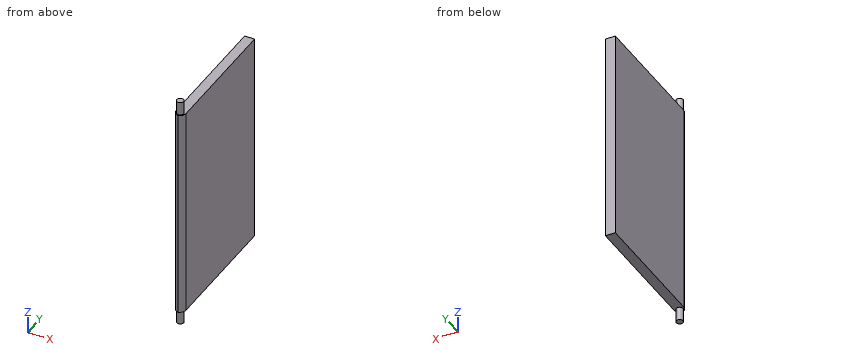
```python
from build123d import *

# Parameters (mm, degrees)
SKETCH1_W           = 101.6
SKETCH1_H           = 64.682803082
BOSS_EXTRUDE1_DEPTH = 4.7625
SKETCH2_R           = 1.631191497
BOSS_EXTRUDE2_DEPTH = 6.35
FILLET2_R           = 3.175


with BuildPart() as part:
    # Sketch1 → Boss-Extrude1 (new body)
    with BuildSketch(Plane(origin=(0, 0, 0), x_dir=(0, 0, -1), z_dir=(1, 0, 0))):
        with Locations((0, 26.994954374)):
            Rectangle(SKETCH1_W, SKETCH1_H)
    extrude(amount=-BOSS_EXTRUDE1_DEPTH)

    # Sketch2 → Boss-Extrude2 (add)
    with BuildSketch(Plane.XY.offset(50.8)):
        with Locations((-2.38125, -2.965197167)):
            Circle(SKETCH2_R)
    boss_extrude2 = extrude(amount=BOSS_EXTRUDE2_DEPTH)

    # Mirror1: Boss-Extrude2 across plane
    add(boss_extrude2.mirror(Plane.XY))

    # Fillet2
    # the kernel refuses this fillet: 3.175 mm, written as the material it takes off along each edge
    with BuildSketch(Plane(origin=(0, -5.346447167, 58.7375), x_dir=(0, 1, 0), z_dir=(0, 0, -1))) as fillet2_piece_1:
        with BuildLine():
            CenterArc((FILLET2_R, -FILLET2_R), FILLET2_R, 90, 90)
            Line((0, -FILLET2_R), (0, 0))
            Line((0, 0), (FILLET2_R, 0))
        make_face()
    extrude(amount=117.475, mode=Mode.SUBTRACT)
    with BuildSketch(Plane(origin=(-4.7625, -5.346447167, 58.7375), x_dir=(0, 1, 0), z_dir=(0, 0, -1))) as fillet2_piece_2:
        with BuildLine():
            CenterArc((FILLET2_R, FILLET2_R), FILLET2_R, 180, 90)
            Line((0, FILLET2_R), (0, 0))
            Line((0, 0), (FILLET2_R, 0))
        make_face()
    extrude(amount=117.475, mode=Mode.SUBTRACT)


solid = part.part
```
Could you check a few things on this model? Use its own coordinates, in mm. Give positions to 0.01 mm unless a question says otherwise; leave off trailing zeros. Order: outer loops, then holes, each group sorted by start corner. A loop starts at its lowest first (then second) coordinate and runs counter-clockwise, first axis right, second up.
Q1. Suppose I cut it at A-A, the plane y = 25. Write out the boundary of the cut face in (x, z).
Q2. Suppose I cut it at B-B, the plane x = -3.1. Write out the boundary of the cut face in (y, z).
Q3. I'm going to push a flat-ended pin straight in: P1, Ø1.5, axis at x = -2, y = 47.5, coming from the -Z side. Where does the tip first touch, or does it pass through?
Q4. If I drill on line 1 along Z through (x, y) = (-1.9, 48.5); line 2 along Y through (x, z) = (-2.3, -33.5); line 3 along Y through (x, z) = (-3.7, 8), over which ranges is the centre line in solid material (lowest first)?
Solution:
1. outline: (-4.76, -50.8) - (0, -50.8) - (0, 50.8) - (-4.76, 50.8) - close
2. outline: (-4.96, -50.8) - (-4.43, -50.8) - (-4.43, -57.15) - (-1.5, -57.15) - (-1.5, -50.8) - (59.34, -50.8) - (59.34, 50.8) - (-1.5, 50.8) - (-1.5, 57.15) - (-4.43, 57.15) - (-4.43, 50.8) - (-4.96, 50.8) - close
3. P1: stops at z = -50.8
4. line 1: z = -50.8 to 50.8
4. line 2: y = -5.22 to 59.34
4. line 3: y = -4.54 to 59.34
